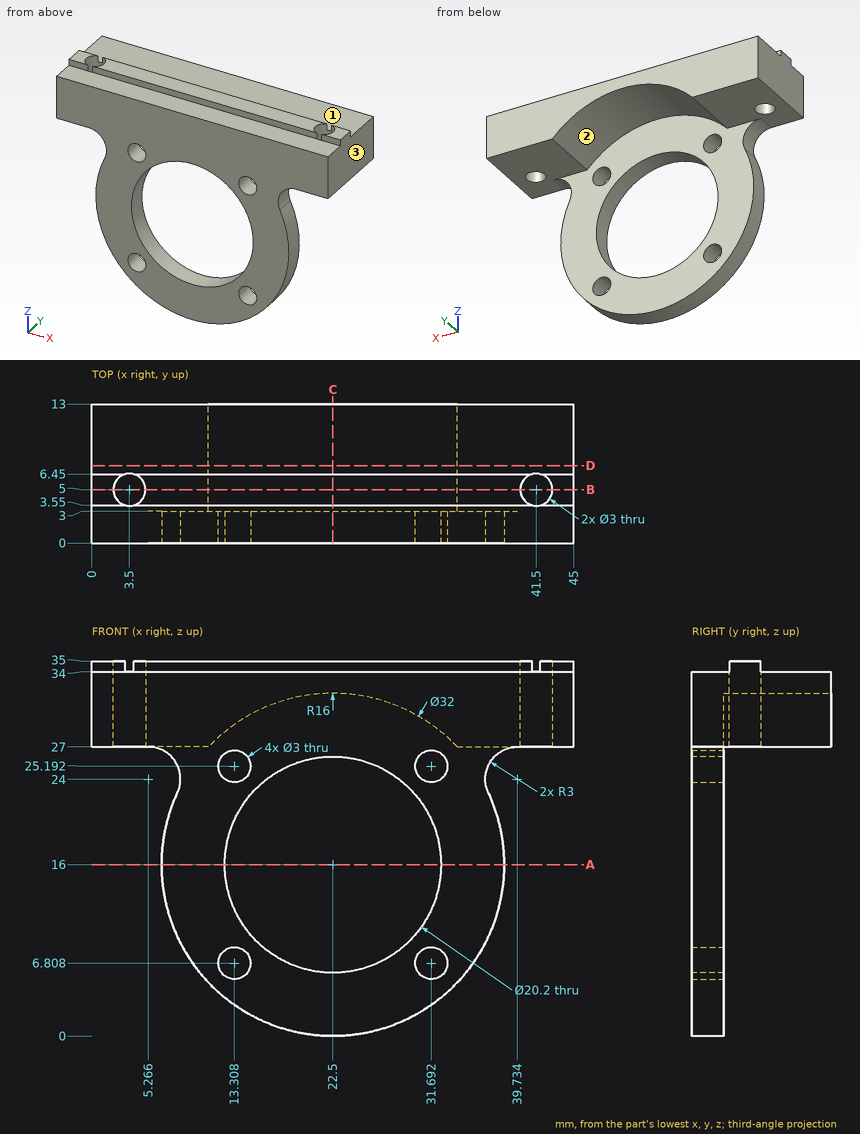
Part print with two shaded views. Sizes in mm from the minimum x, y, z corner. Coordinates: 2 decimals unless noted, no trailing zeros. Order: outer loops, then holes, each group sorted by start corner. A loop starts at its lowest first (then second) coordinate and runs counter-clockwise, first axis right, second up. Notation, with made-up numbers: M 23,-26 L 27,-26 A18 ccw 27,1 Z; hole C 5,-14 d7. An arc over 180 degrees is marked long. Use a Markdown table: item, result.
(1) Flat gauge pins, fed straight in: pin 1 (5 mm diameter, centred on x = 13.31, z = 25.19, fed in from +Y); pin 2 (2.5 mm diameter, centred on x = 3.5, y = 5, fed in from -Z); pin 3 (3 mm diameter, centred on x = 20, y = 1.5, fed in from +Z); pin 4 (1 mm diameter, centred on y = 2.5, z = 6, fed in from -X) (1 decimal). Where does each tip first touch, or does it go through?
A:
| item | result |
|---|---|
| pin 1 | stops at y = 3 |
| pin 2 | passes through |
| pin 3 | stops at z = 34 |
| pin 4 | stops at x = 9.6 |
(2) Pull direction X, two halves, no side cores. Call the marked faces 1, 2 and 3: released by +X, released by -X, zero draft, split by the parting line, or undercut.
A:
| item | result |
|---|---|
| face 1 | zero draft |
| face 2 | undercut |
| face 3 | released by +X |
(3) Cut at A-A on z = 16. Write the cut outline in (x, y).
A:
| item | result |
|---|---|
| outline | M 6.5,0 L 12.4,0 L 12.4,3 L 6.5,3 Z; M 32.6,0 L 38.5,0 L 38.5,3 L 32.6,3 Z |
(4) Cut at D-D on y = 7.25. Write the cut outline in (x, z).
A:
| item | result |
|---|---|
| outline | M 0,27 L 10.88,27 A16 cw 34.12,27 L 45,27 L 45,34 L 0,34 Z |
(5) Probe L1, parallel to Y at x = 9.5, z = 23; L2, parallel to X at y = 2.5, z = 20 (1 decimal); L3, parallel to X at y = 10, z = 29.5 (1 decimal). List the from-to ranges inside material, lowest first.
A:
| item | result |
|---|---|
| L1 | y = 0 to 3 |
| L2 | x = 7 to 13.2, 31.8 to 38 |
| L3 | x = 0 to 13.9, 31.1 to 45 |
(6) Cut at C-C on x = 22.5. Write the cut outline in (y, z), then the cut area to 3 significant figures.
A:
| item | result |
|---|---|
| outline | M 0,0 L 3,0 L 3,5.9 L 0,5.9 Z; M 0,26.1 L 3,26.1 L 3,32 L 13,32 L 13,34 L 6.45,34 L 6.45,35 L 3.55,35 L 3.55,34 L 0,34 Z |
| area | 64.3 mm^2 |
(7) Cut at B-B on y = 5. Write the cut outline in (x, z), then the cut area to 3 significant figures.
A:
| item | result |
|---|---|
| outline | M 0,27 L 2,27 L 2,35 L 0,35 Z; M 5,27 L 10.88,27 A16 cw 34.12,27 L 40,27 L 40,35 L 5,35 Z; M 43,27 L 45,27 L 45,35 L 43,35 Z |
| area | 232 mm^2 |
